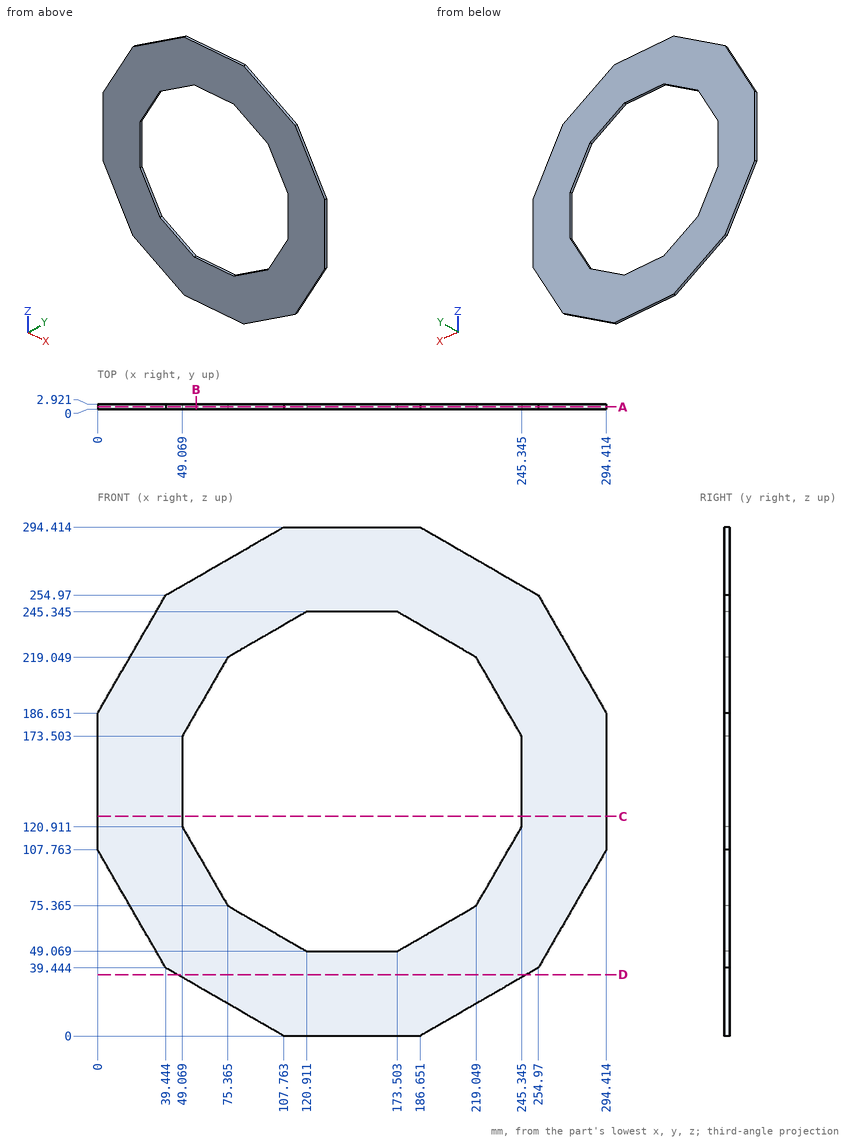
Geometry check sheet. Reference: drawing and pictorial views, mm from the part's lowest x, y, z. Round coordinates to 2 decimals unless told otherwise and drop trailing zeros. Loops run counter-clockwise (first coordinate to the right, second up) from the corner with the lowest first, then second, coordinate; pieces in that order, holes last. Notation, with made-up numbers: (-8, -27.75) - (45, -27.75) arc R23 ccw to (45, -0.75) - close; hole circle Ø8 at (44.25, -7.75). An arc over 180 degrees is marked (long way). Answer in a Markdown table with one row per item. Add a question column.
Q1. Section check A-A on y = 1.3. Enter the section's corners in (x, z) (1 decimal).
Q2. Section check D-D on z = 35.5. Enter the section's corners in (x, y) (1 decimal).
Q3. Material ranges on line 1 (X direction, y = 0.55, z = 172) (1 decimal); line 2 (Z direction, x = 76, y = 2.5) (1 decimal), recorded low to high.
Q4. Section check C-C on z = 127. Enter the section's corners in (x, y) (1 decimal), plus the area to 3 significant figures.
Q5. Section check B-B on x = 57. Enter the section's corners in (y, z).
Found:
| question | item | result |
|---|---|---|
| 1 | outline | (0, 107.8) - (39.4, 39.4) - (107.8, 0) - (186.7, 0) - (255, 39.4) - (294.4, 107.8) - (294.4, 186.7) - (255, 255) - (186.7, 294.4) - (107.8, 294.4) - (39.4, 255) - (0, 186.7) - close; hole (49.1, 120.9) - (75.4, 75.4) - (120.9, 49.1) - (173.5, 49.1) - (219, 75.4) - (245.3, 120.9) - (245.3, 173.5) - (219, 219) - (173.5, 245.3) - (120.9, 245.3) - (75.4, 219) - (49.1, 173.5) - close |
| 2 | outline | (46.3, 0) - (248.1, 0) - (248.1, 2.9) - (46.3, 2.9) - close |
| 3 | line 1 | x = 0 to 49.1, 245.3 to 294.4 |
| 3 | line 2 | z = 18.3 to 75, 219.4 to 276.1 |
| 4 | outline | (0, 0) - (49.1, 0) - (49.1, 2.9) - (0, 2.9) - close; (245.3, 0) - (294.4, 0) - (294.4, 2.9) - (245.3, 2.9) - close |
| 4 | area | 287 mm² |
| 5 | outline | (0, 29.31) - (2.92, 29.31) - (2.92, 107.17) - (0, 107.17) - close; (0, 187.24) - (2.92, 187.24) - (2.92, 265.11) - (0, 265.11) - close |
